Can you work these out from the model? Positions are in its coordinate system, mm. Coordinates: 2 decimals unless noted, no trailing zeros. Order: outer loops, then holes, each group sorted by start corner. A loop starts at its lowest first (then second) coordinate and runs counter-clockwise, first axis right, second up.
```python
from build123d import *

# Parameters (mm, degrees)
SKETCH_1_W          = 30
SKETCH_1_H          = 50
EXTRUDE_1_DEPTH     = 5
SKETCH_3_R          = 1.65
CUT_EXTRUDE_1_DEPTH = 59.523499554
SKETCH_4_W          = 41.234400122
SKETCH_4_H          = 9.68197476
SKETCH_4_W_2        = 47.672667602
SKETCH_4_H_2        = 11.058093
CUT_EXTRUDE_2_DEPTH = 59.523499554
SKETCH_5_W          = 20.505917257
SKETCH_5_H          = 40.348212596
CUT_EXTRUDE_3_DEPTH = 53.668776329
CHAMFER_1_SIZE      = 2


with BuildPart() as part:
    # 草图1 → 凸台-拉伸1 (new body)
    with BuildSketch(Plane(origin=(0, 0, 0), x_dir=(1, 0, 0), z_dir=(0, 1, 0))):
        with Locations((15, -25)):
            Rectangle(SKETCH_1_W, SKETCH_1_H)
    extrude(amount=EXTRUDE_1_DEPTH)

    # 草图2 → 切除-旋转1 (revolve, cut)
    with BuildSketch(Plane(origin=(0, 6.5, 0), x_dir=(1, 0, 0), z_dir=(0, 1, 0))):
        with BuildLine():
            Line((4.95, -25), (25.05, -25))
            ThreePointArc((25.05, -25), (15, -35.05), (4.95, -25))
        make_face()
    revolve(axis=Axis((4.95, 6.5, 25), (1, 0, 0)), mode=Mode.SUBTRACT)

    # 草图3 → 切除-拉伸1 (cut, through all)
    with BuildSketch(Plane(origin=(0, 0, 0), x_dir=(-1, 0, 0), z_dir=(0, -1, 0))):
        with Locations(Location((-8, -37, 0), (0, 0, 90))):
            Circle(SKETCH_3_R)
        with Locations(Location((-22, -37, 0), (0, 0, 90))):
            Circle(SKETCH_3_R)
        with Locations(Location((-8, -13, 0), (0, 0, 90))):
            Circle(SKETCH_3_R)
        with Locations(Location((-22, -13, 0), (0, 0, 90))):
            Circle(SKETCH_3_R)
    extrude(amount=-CUT_EXTRUDE_1_DEPTH, mode=Mode.SUBTRACT)

    # 草图4 → 切除-拉伸2 (cut, through all)
    with BuildSketch(Plane(origin=(0, 5, 0), x_dir=(1, 0, 0), z_dir=(0, 1, 0))):
        with Locations((14.53310274, -2.15901262)):
            Rectangle(SKETCH_4_W, SKETCH_4_H)
        with Locations((15.58976496, -48.5290465)):
            Rectangle(SKETCH_4_W_2, SKETCH_4_H_2)
    extrude(amount=-CUT_EXTRUDE_2_DEPTH, mode=Mode.SUBTRACT)

    # 草图5 → 切除-拉伸3 (cut, through all)
    with BuildSketch(Plane(origin=(0, 5, 0), x_dir=(1, 0, 0), z_dir=(0, 1, 0))):
        with Locations((25.252958629, -25.047535921)):
            Rectangle(SKETCH_5_W, SKETCH_5_H)
    extrude(amount=-CUT_EXTRUDE_3_DEPTH, mode=Mode.SUBTRACT)

    # 倒角1
    chamfer_1_edges = [part.edges().sort_by_distance(p)[0] for p in [
        (0, 0, 25),
        (7.5, 0, 7),
        (7.5, 0, 43),
    ]]
    chamfer(chamfer_1_edges, length=CHAMFER_1_SIZE)


solid = part.part
```
1. Imagine slicing it at D-D on x = 11.75. Please give me the cut outline in (y, z).
Completed:
outline: (0, 9) - (2, 7) - (5, 7) - (5, 15.61) arc R9.51 cw to (0, 18.06) - close; (0, 31.94) arc R9.51 cw to (5, 34.39) - (5, 43) - (2, 43) - (0, 41) - close
2. Please list where these lines run through material, in increasing order: probe 1 along X at (y, z) = (2.3, 37); probe 2 along Z at (x, y) = (7.5, 1.7); probe 3 along X at (y, z) = (1.4, 13).
Completed:
probe 1: x = 0 to 6.35, 9.65 to 15
probe 2: z = 7.3 to 11.43, 14.57 to 20.34, 29.66 to 35.43, 38.57 to 42.7
probe 3: x = 0.6 to 6.35, 9.65 to 15
3. Thinking about a two-plate mould opening in Z: for faces 1 (the flat face through (0, 3, 25)), 2 (the cylindrical face through (8.496, 2.465, 11.426)), 3 (the cylindrical face through (8.07, 2.46, 38.65)), 4 (the flat face through (7, 4, 7)), which applies, pulls with the +Z half, pulls with the -Z half, needs draft (parallel to the pull), parting line crosses it, or undercut?
Completed:
face 1: needs draft
face 2: undercut
face 3: undercut
face 4: pulls with the -Z half
4. Imagine slicing it at B-B on x = 8. Please give me the cut outline in (y, z), then the cut area to 3 significant figures.
Completed:
outline: (0, 9) - (2, 7) - (5, 7) - (5, 11.35) - (0, 11.35) - close; (0, 14.65) - (5, 14.65) - (5, 17.95) arc R7.21 cw to (0, 21.88) - close; (0, 28.12) arc R7.21 cw to (5, 32.05) - (5, 35.35) - (0, 35.35) - close; (0, 38.65) - (5, 38.65) - (5, 43) - (2, 43) - (0, 41) - close
area: 85.8 mm2
5. Imagine slicing it at A-A on z = 37. Please give me the cut outline in (x, y).
Completed:
outline: (0, 2) - (2, 0) - (6.35, 0) - (6.35, 5) - (0, 5) - close; (9.65, 0) - (15, 0) - (15, 5) - (9.65, 5) - close
6. Imagine slicing it at C-C on y = 3.65. Please give me the cut outline in (x, z).
Completed:
outline: (0, 7) - (15, 7) - (15, 15.36) arc R9.64 cw to (15, 34.64) - (15, 43) - (0, 43) - close; hole circle Ø3.3 at (8, 13); hole circle Ø3.3 at (8, 37)
